```python
from build123d import *

# Parameters (mm, degrees)
SKETCH1_W           = 27.94
SKETCH1_H           = 17.78
SKETCH1_W_2         = 2.54
SKETCH1_H_2         = 12.7
BOSS_EXTRUDE2_DEPTH = 2.54
SKETCH3_R           = 1.27
BOSS_EXTRUDE3_DEPTH = 3.302
SKETCH6_W           = 2.503557337
SKETCH6_H           = 12.554229347
BOSS_EXTRUDE6_DEPTH = 3.302


with BuildPart() as part:
    # Sketch1 → Boss-Extrude2 (new body)
    with BuildSketch(Plane(origin=(0, 0, 0), x_dir=(1, 0, 0), z_dir=(0, 1, 0))):
        Rectangle(SKETCH1_W, SKETCH1_H)
        with Locations((-10.20489899, 0)):
            Rectangle(SKETCH1_W_2, SKETCH1_H_2, mode=Mode.SUBTRACT)
        with Locations((10.20489899, 0)):
            Rectangle(SKETCH1_W_2, SKETCH1_H_2, mode=Mode.SUBTRACT)
    extrude(amount=BOSS_EXTRUDE2_DEPTH)

    # Sketch3 → Boss-Extrude3 (add)
    with BuildSketch(Plane(origin=(0, 2.54, 0), x_dir=(1, 0, 0), z_dir=(0, 1, 0))):
        with Locations(Location((-5.318941048, 2.54, 0), (0, 0, 90))):
            Circle(SKETCH3_R)
        with Locations(Location((5.318941048, 2.54, 0), (0, 0, 90))):
            Circle(SKETCH3_R)
    extrude(amount=BOSS_EXTRUDE3_DEPTH)

    # Sketch6 → Boss-Extrude6 (add)
    with BuildSketch(Plane(origin=(0, 2.54, 0), x_dir=(1, 0, 0), z_dir=(0, 1, 0))):
        Polygon((-7.215647318, 4.760339872), (7.384221332, 4.760339872), (7.384221332, -8.817114674), (13.988221332, -8.817114674), (13.97, 8.89), (-13.97, 8.89), (-13.97, -8.89), (-7.347778668, -8.89), align=None)
        with Locations((10.223120322, 0.072885327)):
            Rectangle(SKETCH6_W, SKETCH6_H, mode=Mode.SUBTRACT)
        with Locations((-10.186677659, 0.072885327)):
            Rectangle(SKETCH6_W, SKETCH6_H, mode=Mode.SUBTRACT)
    extrude(amount=BOSS_EXTRUDE6_DEPTH)


solid = part.part
```
Design review of the part built by this model. Coordinates are the model's own, in mm. A direction names the side the tool comes from. Round coordinates to 2 decimals unless told otherwise and drop trailing zeros. Write each loop counter-clockwise with the first axis right and the second up, starting at its lowest first coordinate (ties: lowest second). Pieces come first, ordered by that corner, then holes.
Item 1: We need section B-B on y = 4.3. Write out the cut boundary in (x, z), and give its area (3 significant figures).
Item 2: The part is to be moulded in two halves that separate along X. For faces 1 (the flat face through (11, 4, 8.817)), 2 (the flat face through (-13.97, 3, 0)), 3 (the flat face through (-10, 4, 6.204)), say which applies: +X half, -X half, draft (parallel to the pull), parting line (faces both ways), or undercut.
Item 3: We need section C-C on z = -3.5. State how many separate pieces and enclosed holes the cut face has, and give its area (3 significant figures).
Item 4: Clearance check with flat-ended pins moving along their axes: pin 1 Ø6 at (x, z) = (-7, -3) entering from -Y; pin 2 Ø3 at (y, z) = (4, -3.5) entering from +X; pin 3 Ø1 at (x, y) = (-1, 5) entering from +Z. State where each tip first meets the part, or that it passes through.
Item 5: For faces 4 (the cylindrical face through (6.559, 4.168, -2.265)), 5 (the flat face through (10, 4, 6.204)), 6 (the flat face through (7.384, 4, 2)), 7 (the flat face through (10, 1, 6.35)), 8 (the flat face through (5, 5.842, -3)), list the 3-axis set-ups (+Z, -Z, +X, -X, +Y, -Y) from which the entire face can be reached by the end or side of a thin tool; tool diameter is ignored.
Item 6: We need section A-A on x = 10.25. Write out the cut boundary in (y, z).
Item 7: We need section D-D on y = 1.6. Write out the cut boundary in (x, z), and give its area (3 significant figures).
Item 8: For probe 1 along X at (y, z) = (1.7, 2.25); probe 2 along X at (y, z) = (5.15, -6); probe 3 along Z at (x, y) = (-9, 5), list the stretches that pass through material, from the lowest coordinate up.
Returned:
1. outline: (-13.97, -8.89) - (13.97, -8.89) - (13.99, 8.82) - (7.38, 8.82) - (7.38, -4.76) - (-7.22, -4.76) - (-7.35, 8.89) - (-13.97, 8.89) - close; circle Ø2.54 at (-5.32, -2.54); circle Ø2.54 at (5.32, -2.54); hole (-11.44, -6.35) - (-8.93, -6.35) - (-8.93, 6.2) - (-11.44, 6.2) - close; hole (8.97, -6.35) - (11.47, -6.35) - (11.47, 6.2) - (8.97, 6.2) - close
1. area: 244 mm2
2. face 1: draft
2. face 2: -X half
2. face 3: undercut
3. separate pieces: 3
3. enclosed holes: 0
3. area: 96.5 mm2
4. pin 1: stops at y = 0
4. pin 2: stops at x = 13.98
4. pin 3: stops at z = -4.76
5. face 4: +Y
5. face 5: +Y, -Y
5. face 6: +Z, +Y
5. face 7: -Y
5. face 8: +Z, -Z, +X, -X, +Y
6. outline: (0, -8.89) - (5.84, -8.89) - (5.84, -6.35) - (0, -6.35) - close; (0, 6.35) - (2.54, 6.35) - (2.54, 6.2) - (5.84, 6.2) - (5.84, 8.82) - (2.54, 8.82) - (2.54, 8.89) - (0, 8.89) - close
7. outline: (-13.97, -8.89) - (13.97, -8.89) - (13.97, 8.89) - (-13.97, 8.89) - close; hole (-11.47, -6.35) - (-8.93, -6.35) - (-8.93, 6.35) - (-11.47, 6.35) - close; hole (8.93, -6.35) - (11.47, -6.35) - (11.47, 6.35) - (8.93, 6.35) - close
7. area: 432 mm2
8. probe 1: x = -13.97 to -11.47, -8.93 to 8.93, 11.47 to 13.97
8. probe 2: x = -13.97 to -11.44, -8.93 to 8.97, 11.47 to 13.97
8. probe 3: z = -8.89 to -6.35, 6.2 to 8.89
